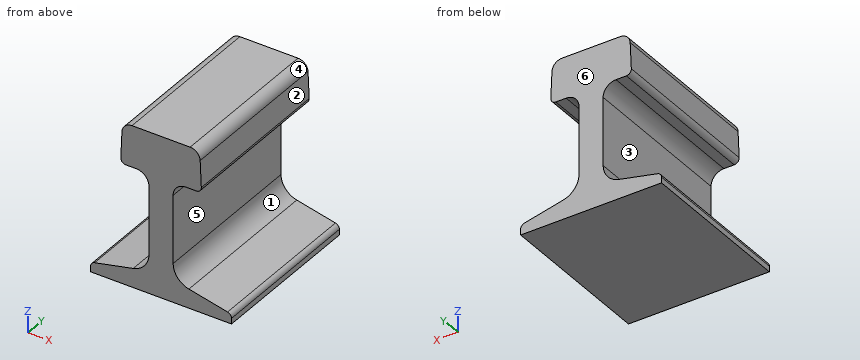
from build123d import *

# Parameters (mm, degrees)
F1_DEPTH = 25.4


with BuildPart() as f1:
    # F0 (on Front) → F1 (new body)
    with BuildSketch(Plane.XZ):
        with BuildLine():
            Line((0, 0.886948), (0, 0))
            Line((0, 0), (22.225, 0))
            Line((22.225, 0), (22.225, 0.886948))
            ThreePointArc((22.225, 0.886948), (22.050283, 1.383775), (21.603049, 1.661883))
            Line((21.603049, 1.661883), (15.505304, 3.013721))
            ThreePointArc((15.505304, 3.013721), (13.716367, 4.126153), (13.0175, 6.113461))
            Line((13.0175, 6.113461), (13.0175, 16.8402))
            ThreePointArc((13.0175, 16.8402), (13.612659, 18.277041), (15.0495, 18.8722))
            Line((15.0495, 18.8722), (16.671438, 18.8722))
            ThreePointArc((16.671438, 18.8722), (17.244814, 19.117062), (17.464432, 19.700573))
            Line((17.464432, 19.700573), (17.281879, 23.881746))
            ThreePointArc((17.281879, 23.881746), (16.793666, 24.959253), (15.695889, 25.4))
            Line((15.695889, 25.4), (6.529111, 25.4))
            ThreePointArc((6.529111, 25.4), (5.431334, 24.959253), (4.943121, 23.881746))
            Line((4.943121, 23.881746), (4.760568, 19.700573))
            ThreePointArc((4.760568, 19.700573), (4.980186, 19.117062), (5.553562, 18.8722))
            Line((5.553562, 18.8722), (7.1755, 18.8722))
            ThreePointArc((7.1755, 18.8722), (8.612341, 18.277041), (9.2075, 16.8402))
            Line((9.2075, 16.8402), (9.2075, 6.113461))
            ThreePointArc((9.2075, 6.113461), (8.508633, 4.126153), (6.719696, 3.013721))
            Line((6.719696, 3.013721), (0.621951, 1.661883))
            ThreePointArc((0.621951, 1.661883), (0.174717, 1.383775), (0, 0.886948))
        make_face()
    extrude(amount=F1_DEPTH)


solid = f1.part
Can you work these out from the model? Positions are in its coordinate system, mm. Face numbers are marked on the shaded views. A direction names the side the tool comes from. Round coordinates to 2 decimals unless told otherwise and drop trailing zeros. Order: outer loops, then holes, each group sorted by start corner. A loop starts at its lowest first (then second) coordinate and runs counter-clockwise, first axis right, second up. Notation, with made-up numbers: M 79.25,6.5 L 110.25,6.5 A18 cw 110.25,36.5 Z; hole C -24.75,-23.75 d3. An arc over 180 degrees is marked long. Use a Markdown table: item, result.
1) Imagine slicing it at A-A (x = 14). List the corners of the cut face in (y, z) for me.
Geometry says:
| item | result |
|---|---|
| outline | M -25.4,0 L 0,0 L 0,3.82 L -25.4,3.82 Z; M -25.4,18.58 L 0,18.58 L 0,25.4 L -25.4,25.4 Z |
2) On a 3-axis mill with a long thin cutter (end or side, diameter ignored), from which of +Z, -Z, +X, -X, +Y, -Y can I reach the whole of each face in a straight line? I mean the marked faces 1, 2 and 3. Say none if no direction works.
Geometry says:
| item | result |
|---|---|
| face 1 | +X, +Y, -Y |
| face 2 | +Z, +X, +Y, -Y |
| face 3 | -X, +Y, -Y |
3) If I drill on line 1 along X through (y, z) = (-8, 23.75); line 2 along Z through (x, y) = (15, -3.25); line 3 along X through (y, z) = (-9.5, 13), over which ranges is the centre line in solid material (lowest first)?
Geometry says:
| item | result |
|---|---|
| line 1 | x = 4.94 to 17.29 |
| line 2 | z = 0 to 3.17, 18.87 to 25.4 |
| line 3 | x = 9.21 to 13.02 |
4) If we mould it in two halves opening along Z, with no side actions, what happens to the marked faces 4, 5 and 6? For each: +Z half, -Z half, draft (parallel to the pull), parting line (faces both ways), or undercut.
Geometry says:
| item | result |
|---|---|
| face 4 | +Z half |
| face 5 | undercut |
| face 6 | draft |
5) Imagine slicing it at D-D (x = 18.75). List the corners of the cut face in (y, z) for me.
Geometry says:
| item | result |
|---|---|
| outline | M -25.4,0 L 0,0 L 0,2.29 L -25.4,2.29 Z |
6) I'm going to push flat-ended pins straight in: P1, Ø8.5, axis at y = -12, z = 14, coming from the -X side; P2, Ø5.5, axis at y = -14, z = 10.5, coming from the +X side; P3, Ø12, axis at y = -6, z = 19.5, coming from the -X side. Where does each tip first touch, or does it pass through?
Geometry says:
| item | result |
|---|---|
| P1 | stops at x = 8.64 |
| P2 | stops at x = 13.02 |
| P3 | stops at x = 4.76 |
7) Imagine slicing it at C-C (z = 7.25). List the corners of the cut face in (x, y) for me.
Geometry says:
| item | result |
|---|---|
| outline | M 9.21,-25.4 L 13.02,-25.4 L 13.02,0 L 9.21,0 Z |
